Verification items for the finished model (mm, model axes). A direction names the side the tool comes from. Round coordinates to 2 decimals unless told otherwise and drop trailing zeros. Write each loop counter-clockwise with the first axis right and the second up, starting at its lowest first coordinate (ties: lowest second). Pieces come first, ordered by that corner, then holes. Notation, with made-up numbers: M 32.5,15.5 L 69.5,15.5 A18 ccw 69.5,26.5 Z; hole C -32,-24 d11. An arc over 180 degrees is marked long. One line per item, written item: value. Start each with the question number.
Item 1: Section check A-A, the plane y = 154.5. Record the cut outline in (x, z), then the cut area to 3 significant figures.
Item 2: Thickness scan on probe 1 along Y at (x, z) = (56.65, -8.85); probe 2 along Z at (x, y) = (56, 259); probe 3 along X at (y, z) = (80, -6). Record the ranges inside material, lowest first. Write a range as from..to.
Item 3: Tool access check on faces 1 (the face through (55, 82, -6)), 2 (the face through (0, 170, -1)). Record the directions out of +Z, -Z, +X, -X, +Y, -Y that give a thin tool (end or side, any length) a straight path to the whole face; none if there is none.
Item 4: Gauge pin test, flat ends, axial feed: pin 1 (0.6 mm diameter, centred on x = 56.5, z = -6.5, fed in from -Y); pin 2 (3.5 mm diameter, centred on y = 259.5, z = -8.85, fed in from -X); pin 3 (2 mm diameter, centred on x = 39, y = 127.5, fed in from +Z); pin 4 (2 mm diameter, centred on x = 0.5, z = -7.5, fed in from +Y). Record the tip position at first contact, or that the pin passes through.
Item 5: Draft check along X on faces 3 (the face through (57, 170, -1)), 4 (the face through (2, 259, -6)), 5 (the face through (29, 169, 0)). Enter one of: +X half, -X half, draft (parallel to the pull), parting line (faces both ways), or undercut.
Item 6: Section check B-B, the plane x = 48.5. Record the cut outline in (y, z).
from build123d import *

# Parameters (mm, degrees)
DODANIE_WYCI_GNI_CIE1_DEPTH = 342
SZKIC3_W                    = 2
SZKIC3_H                    = 15
DODANIE_WYCI_GNI_CIE2_DEPTH = 12
SZKIC4_R                    = 2
WYTNIJ_WYCI_GNI_CIE1_DEPTH  = 10
SZKIC5_R                    = 2
WYTNIJ_WYCI_GNI_CIE2_DEPTH  = 10


with BuildPart() as part:
    # Szkic1 → Dodanie-wyciągnięcie1 (new body)
    with BuildSketch(Plane(origin=(0, 0, 0), x_dir=(1, 0, 0), z_dir=(0, 1, 0))):
        Polygon((0, 0), (0, 1.85), (24, 1.85), (24, 31.85), (24.5, 31.85), (24.5, 2.35), (35, 2.35), (35, 1.85), (57, 1.85), (57, 0), align=None)
    extrude(amount=DODANIE_WYCI_GNI_CIE1_DEPTH)

    # Szkic3 → Dodanie-wyciągnięcie2 (add)
    with BuildSketch(Plane(origin=(0, 0, -1.85), x_dir=(-1, 0, 0), z_dir=(0, 0, -1))):
        with Locations((-56, 82.5)):
            Rectangle(SZKIC3_W, SZKIC3_H)
        with Locations((-56, 259.5)):
            Rectangle(SZKIC3_W, SZKIC3_H)
        with Locations((-1, 82.5)):
            Rectangle(SZKIC3_W, SZKIC3_H)
        with Locations((-1, 259.5)):
            Rectangle(SZKIC3_W, SZKIC3_H)
    extrude(amount=DODANIE_WYCI_GNI_CIE2_DEPTH)

    # Szkic4 → Wytnij-wyciągnięcie1 (cut)
    with BuildSketch(Plane.ZY):
        with Locations((-8.85, 82.5)):
            Circle(SZKIC4_R)
        with Locations((-8.85, 259.5)):
            Circle(SZKIC4_R)
    extrude(amount=-WYTNIJ_WYCI_GNI_CIE1_DEPTH, mode=Mode.SUBTRACT)

    # Szkic5 → Wytnij-wyciągnięcie2 (cut)
    with BuildSketch(Plane(origin=(57, 0, 0), x_dir=(0, 0, -1), z_dir=(1, 0, 0))):
        with Locations((8.85, 259.5)):
            Circle(SZKIC5_R)
        with Locations((8.85, 82.5)):
            Circle(SZKIC5_R)
    extrude(amount=-WYTNIJ_WYCI_GNI_CIE2_DEPTH, mode=Mode.SUBTRACT)


solid = part.part
Response values:
1. outline: M 0,-1.85 L 24,-1.85 L 24,-31.85 L 24.5,-31.85 L 24.5,-2.35 L 35,-2.35 L 35,-1.85 L 57,-1.85 L 57,0 L 0,0 Z
1. area: 126 mm2
2. probe 1: y = 75..80.5, 84.5..90, 252..257.5, 261.5..267
2. probe 2: z = -13.85..-10.79, -6.91..0
2. probe 3: x = 0..2, 24..24.5, 55..57
3. face 1: -Z, +Y, -Y
3. face 2: +Z, -Z, -X, +Y, -Y
4. pin 1: stops at y = 75
4. pin 2: stops at x = 24
4. pin 3: stops at z = 0
4. pin 4: stops at y = 267
5. face 3: +X half
5. face 4: undercut
5. face 5: draft
6. outline: M 0,-1.85 L 342,-1.85 L 342,0 L 0,0 Z
